Input: dimensioned drawing with shaded views. Units: mm. Origin: part minimum x, y, z. A direction names the side the tool comes from. Round coordinates to 2 decimals unless told otherwise and drop trailing zeros. Order: outer loops, then holes, each group sorted by start corner. A loop starts at its lowest first (then second) coordinate and runs counter-clockwise, first axis right, second up. Notation, with made-up numbers: (80, 85) - (91, 85) arc R12 ccw to (91, 99) - close; hole circle Ø5 at (48.25, 7). An arc over 180 degrees is marked (long way). Return JSON: item names as keys, results as strings. Group by question number.
1) Contact query for flat-ended pins moving along their axis: P1, Ø1, axis at x = 29, y = 7.5, coming from the +Z side; P2, Ø1, axis at y = 7.5, z = 23, coming from the +X side; P3, Ø1, axis at x = 24, y = 2.5, coming from the +Z side. Output: stop coordinate, or through.
2) Access query for the marked faces 1 and 2. Directions: +Z, -Z, +X, -X, +Y, -Y. A direction counts if a zero-diameter tool reaches every point of the face in a straight line with its end or side. Return the directions, or none.
3) Section D-D, the plane z = 4.5. Return loops of the section in (x, y), plus the area to 3 significant figures.
4) Section B-B, the plane y = 19. Return loops of the section in (x, z).
5) Section A-A, the plane z = 27. Return loops of the section in (x, y), plus the area to 3 significant figures.
6) Ray query, line 1 (Z direction, x = 26, y = 16.5); line 2 (X direction, y = 10.25, z = 4). Return the intervals inside material, ascending. Write a range as from..to.
7) Section C-C, the plane x = 15. Return loops of the section in (y, z).
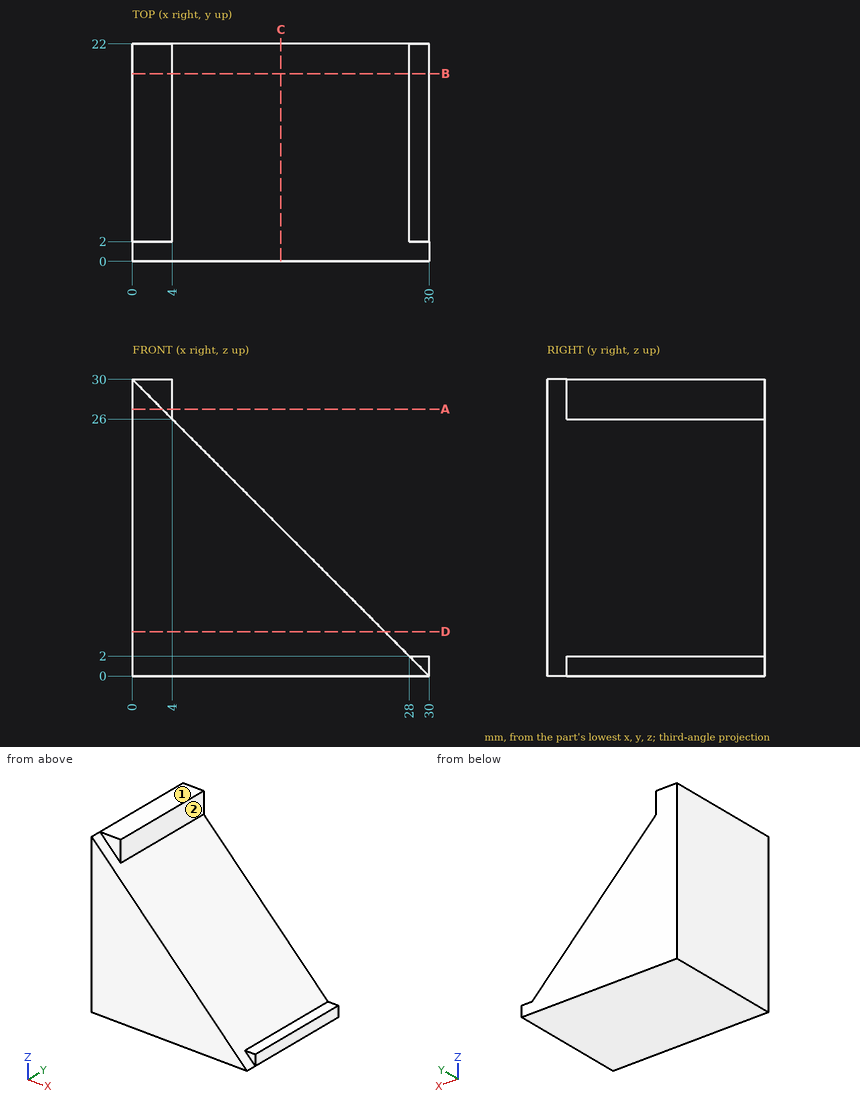
Geometry check:
{
 "1": {"P1": "z = 2", "P2": "x = 7.5", "P3": "z = 6.5"},
 "2": {"face 1": "+Z, +X, -X, +Y, -Y", "face 2": "+Z, +X, +Y, -Y"},
 "3": {"outline": "(0, 0) - (25.5, 0) - (25.5, 22) - (0, 22) - close", "area": "561 mm2"},
 "4": {"outline": "(0, 0) - (30, 0) - (30, 2) - (28, 2) - (4, 26) - (4, 30) - (0, 30) - close"},
 "5": {"outline": "(0, 0) - (3, 0) - (3, 2) - (4, 2) - (4, 22) - (0, 22) - close", "area": "86.0 mm2"},
 "6": {"line 1": "0..4", "line 2": "0..26"},
 "7": {"outline": "(0, 0) - (22, 0) - (22, 15) - (0, 15) - close"}
}
